Part model, mm, in its own coordinate system. Coordinates: 2 decimals unless noted, no trailing zeros. Write each loop counter-clockwise with the first axis right and the second up, starting at its lowest first coordinate (ties: lowest second). Pieces come first, ordered by that corner, then holes. Notation, with made-up numbers: (51, -14.5) -> (87, -14.5) arc R15 ccw to (87, 1.5) -> close; hole circle Ø4 at (-29.75, 67.25). An arc over 180 degrees is marked (long way). Write item = value, one per line. Start each with the question number.
Q1. Pull direction Y, two halves, no side cores. Call faces 1 (the cylindrical face through (16.2, 1.36, 0.45)), 2 (the flat face through (0, 0, 0)), 3 (the flat face through (0, 22.225, 2)), 4 (the flat face through (0, -22.225, 2)): released by +Y, released by -Y, zero draft, split by the parting line, or undercut.
Q2. Band-saw the part on B-B, the plane z = 2.4. List the corners of the cut face in (x, y) (3 decimals).
Q3. Probe line 1 (Y direction, x = 19.05, z = 0.7) (3 decimals); line 2 (X direction, y = 3, z = 2.05) (3 decimals); line 3 (X direction, y = -1, z = 2.45) (3 decimals). List the from-to ranges inside material, lowest first.
Q4. Band-saw the part on A-A, the plane x = -19.05. List the corners of the cut face in (y, z) (3 decimals).
from build123d import *

# Parameters (mm, degrees)
SKETCH1_W                                    = 69.85
SKETCH1_H                                    = 44.45
BOSS_EXTRUDE1_DEPTH                          = 4.7498
CSK_FOR_1_4_FLAT_HEAD_SOCKET_CAP_SCR_2_COUNT = 2
CSK_FOR_1_4_FLAT_HEAD_SOCKET_CAP_SCR_2_PITCH = 38.1


with BuildPart() as part:
    # Sketch1 → Boss-Extrude1 (new body)
    with BuildSketch(Plane.XY):
        Rectangle(SKETCH1_W, SKETCH1_H)
    extrude(amount=BOSS_EXTRUDE1_DEPTH)

    # Sketch3 → CSK for 1/4 Flat Head Socket Cap Screw1 (revolve, cut)
    with BuildSketch(Plane(origin=(-19.05, 3.175, 4.7498), x_dir=(0, -1, 0), z_dir=(1, 0, 0))):
        Polygon((0, 0), (0, 4.7498), (3.3782, 4.7498), (3.3782, 3.871564875), (6.7437, 0), align=None)
    csk_for_1_4_flat_head_socket_cap_screw1 = revolve(axis=Axis((-19.05, 3.175, 11.0998), (0, 0, -1)), mode=Mode.SUBTRACT)

    # CSK for 1_4 Flat Head Socket Cap Scr 2: CSK for 1/4 Flat Head Socket Cap Screw1 ×2
    with Locations(*[(i * CSK_FOR_1_4_FLAT_HEAD_SOCKET_CAP_SCR_2_PITCH, 0, 0) for i in range(1, CSK_FOR_1_4_FLAT_HEAD_SOCKET_CAP_SCR_2_COUNT)]):
        add(csk_for_1_4_flat_head_socket_cap_screw1, mode=Mode.SUBTRACT)


solid = part.part
Ans:
q1.face_1 = undercut
q1.face_2 = zero draft
q1.face_3 = released by +Y
q1.face_4 = released by -Y
q2.outline = (-34.925, -22.225) -> (34.925, -22.225) -> (34.925, 22.225) -> (-34.925, 22.225) -> close; hole circle Ø9.402 at (-19.05, 3.175); hole circle Ø9.402 at (19.05, 3.175)
q3.line_1 = -22.225 to -0.203, 6.553 to 22.225
q3.line_2 = -34.925 to -23.443, -14.657 to 14.657, 23.443 to 34.925
q3.line_3 = -34.925 to -21.304, -16.796 to 16.796, 21.304 to 34.925
q4.outline = (-22.225, 0) -> (-0.203, 0) -> (-0.203, 0.878) -> (-3.569, 4.75) -> (-22.225, 4.75) -> close; (6.553, 0) -> (22.225, 0) -> (22.225, 4.75) -> (9.919, 4.75) -> (6.553, 0.878) -> close
